Part print with two shaded views. Sizes in mm from the minimum x, y, z corner. A direction names the side the tool comes from. Coordinates: 2 decimals unless noted, no trailing zeros. Loops run counter-clockwise (first coordinate to the right, second up) from the corner with the lowest first, then second, coordinate; pieces in that order, holes last.
Item 1: Cut at B-B (y = 28.25). List the corners of the cut face in (x, z), and give its area (3 significant figures).
Item 2: Cut at D-D (y = 8.5). List the corners of the cut face in (x, z).
Item 3: Cut at A-A (z = 19.5). List the corners of the cut face in (x, y).
Item 4: Mould opens along Z. For the marked faces 3, 4 and 5 say: released by +Z, released by -Z, zero draft, split by the parting line, or undercut.
Item 5: Cut at C-C (x = 26.25). List the corners of the cut face in (y, z), and give its area (3 significant figures).
Item 6: Drill centre lines: line 1 along Z through (x, y) = (25.5, 5.75); line 2 along X through (y, z) = (3, 30); line 3 along Z through (x, y) = (28, 19.5). Where is each one in solid material? Low to high.
Item 7: Flat gauge pins, fed straight in: pin 1 (15.5 mm diameter, centred on x = 7, z = 36, fed in from +Y); pin 2 (1.6 mm diameter, centred on x = 14, z = 29.5, fed in from -Y). Where does each tip first touch, or does it go through?
Item 8: 3-axis set-ups, long thin cutter, end or side, ignore diameter. For the marked faces 1 and 2: which of +Z, -Z, +X, -X, +Y, -Y reach the whole face in a straight line?
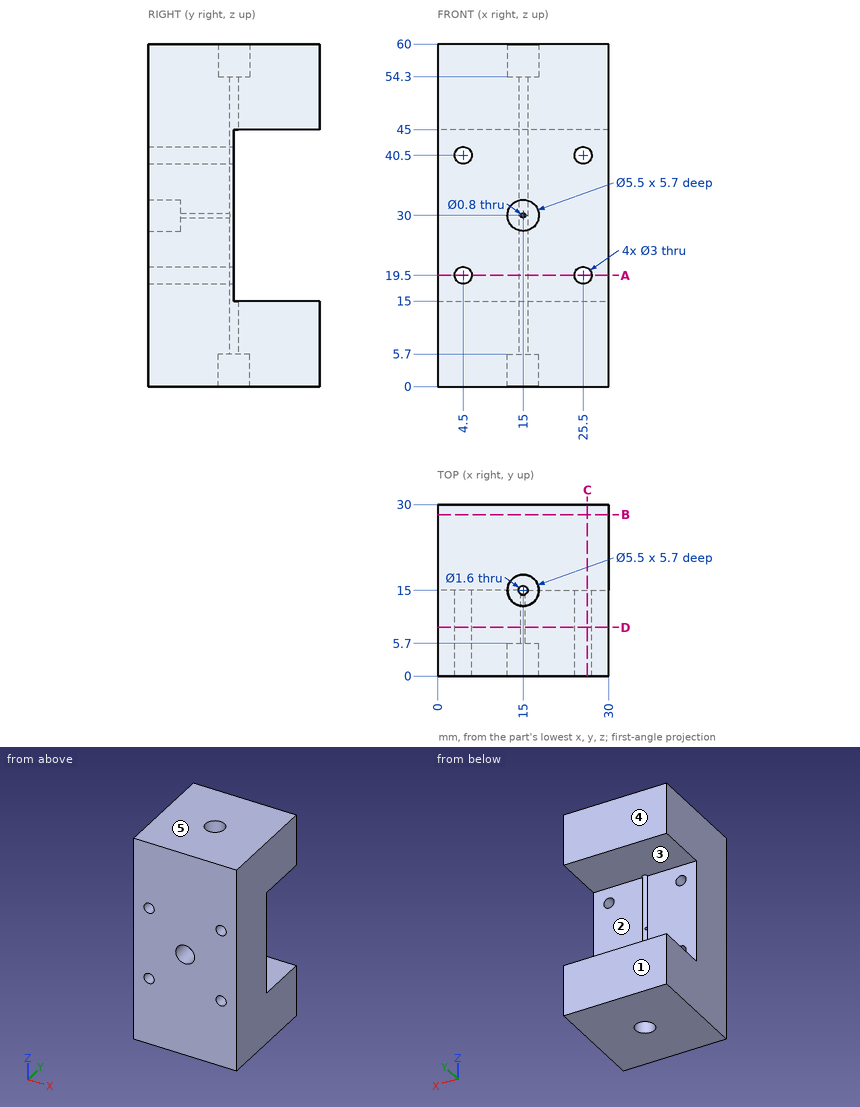
Filled sheet:
1. outline: (0, 0) - (30, 0) - (30, 15) - (0, 15) - close; (0, 45) - (30, 45) - (30, 60) - (0, 60) - close
1. area: 900 mm2
2. outline: (0, 0) - (30, 0) - (30, 60) - (0, 60) - close; hole circle Ø3 at (4.5, 19.5); hole circle Ø3 at (4.5, 40.5); hole circle Ø0.8 at (15, 30); hole circle Ø3 at (25.5, 19.5); hole circle Ø3 at (25.5, 40.5)
3. outline: (0, 0) - (3, 0) - (3, 15) - (0, 15) - close; (6, 0) - (24, 0) - (24, 15) - (15.8, 15) arc R0.8 cw to (14.2, 15) - (6, 15) - close; (27, 0) - (30, 0) - (30, 15) - (27, 15) - close
4. face 3: undercut
4. face 4: zero draft
4. face 5: released by +Z
5. outline: (0, 0) - (30, 0) - (30, 15) - (15, 15) - (15, 18.2) - (0, 18.2) - close; (0, 20.8) - (15, 20.8) - (15, 39.2) - (0, 39.2) - close; (0, 41.8) - (15, 41.8) - (15, 45) - (30, 45) - (30, 60) - (0, 60) - close
5. area: 1,270 mm2
6. line 1: z = 0 to 18, 21 to 39, 42 to 60
6. line 2: x = 0 to 12.25, 17.75 to 30
6. line 3: z = 0 to 15, 45 to 60
7. pin 1: stops at y = 15
7. pin 2: stops at y = 5.7
8. face 1: +Z, -Z, +X, -X, +Y
8. face 2: +X, -X, +Y
